Geometry check sheet. Reference: drawing and pictorial views, mm from the part's lowest x, y, z. A direction names the side the tool comes from. Give positions to 0.01 mm unless a question says otherwise; leave off trailing zeros. Write each loop counter-clockwise with the first axis right and the second up, starting at its lowest first coordinate (ties: lowest second). Pieces come first, ordered by that corner, then holes. Notation, with made-up numbers: M 76,66.5 L 123,66.5 A21 ccw 123,83.5 Z; hole C 20,-9 d11. An arc over 180 degrees is marked long. Write item = value, one per line. Start each with the question number.
1) Mould release check, pull along X, two halves, no side actions. Record for the marked faces 1, 2 and 3: released by +X, released by -X, zero draft, split by the parting line, or undercut.
2) Scan lines: line 1 along Y through (x, z) = (45, 9.1); line 2 along X through (y, z) = (51, 6); line 3 along Z through (x, y) = (38, 16). Record each from-to range of solid material in increasing order. Write a range as [from, to].
3) Go/stop test with flat-tipped pins: pin 1 (3 mm diameter, centred on y = 35, z = 10.5, fed in from -X); pin 2 (3 mm diameter, centred on y = 63.5, z = 3, fed in from -X). Record where each tip stops, or that it passes through.
4) Cross-section at B-B, the plane y = 40. Record the cut outline in (x, z), plus the area to 3 significant figures.
5) Cross-section at A-A, the plane x = 45. Record the cut outline in (y, z), plus the area to 3 significant figures.
6) Cross-section at D-D, the plane y = 11. Record the cut outline in (x, z).
7) Access from +Z, -Z, +X, -X, +Y, -Y to the whole of each face (thin tool, end or side, straight path). Record for the marked faces 4 and 5.
8) Cross-section at C-C, the plane z = 5.25. Record the cut outline in (x, y), plus the area to 3 significant figures.
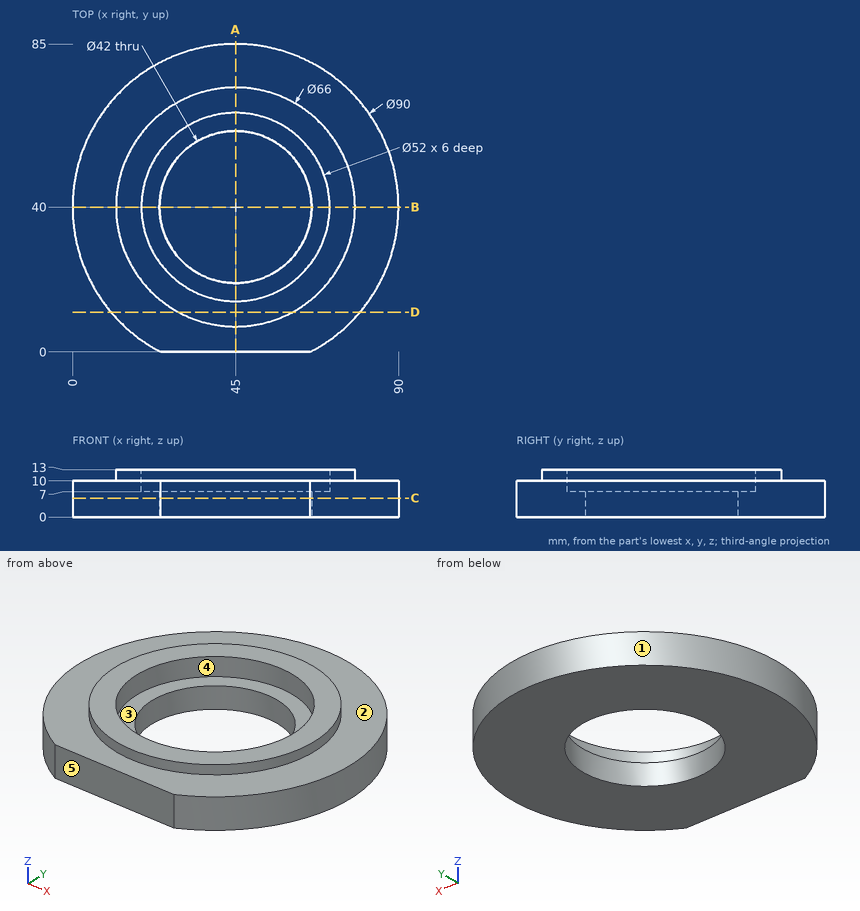
Reply:
q1.face_1 = split by the parting line
q1.face_2 = zero draft
q1.face_3 = undercut
q2.line_1 = [0, 14], [66, 85]
q2.line_2 = [1.37, 27.11], [62.89, 88.63]
q2.line_3 = [0, 7]
q3.pin_1 = 0.14
q3.pin_2 = 5.74
q4.outline = M 0,0 L 24,0 L 24,7 L 19,7 L 19,13 L 12,13 L 12,10 L 0,10 Z; M 66,0 L 90,0 L 90,10 L 78,10 L 78,13 L 71,13 L 71,7 L 66,7 Z
q4.area = 492 mm2
q5.outline = M 0,0 L 19,0 L 19,7 L 14,7 L 14,13 L 7,13 L 7,10 L 0,10 Z; M 61,0 L 85,0 L 85,10 L 73,10 L 73,13 L 66,13 L 66,7 L 61,7 Z
q5.area = 442 mm2
q6.outline = M 10.59,0 L 79.41,0 L 79.41,10 L 60.75,10 L 60.75,13 L 29.25,13 L 29.25,10 L 10.59,10 Z
q7.face_4 = +Z
q7.face_5 = +Z, -Z, +X, -X, -Y
q8.outline = M 24.38,0 L 65.62,0 A45 ccw long Z; hole C 45,40 d42
q8.area = 4,840 mm2
